Could you check a few things on this drawing? It's one solid part, dimensions in mm from its lowest x, y, z. A direction names the side the tool comes from. Round coordinates to 2 decimals unless told otherwise and drop trailing zeros. Loops run counter-clockwise (first coordinate to the right, second up) from the corner with the lowest first, then second, coordinate; pieces in that order, holes last. Notation, with made-up numbers: (81.5, -11) -> (118.5, -11) arc R31 cw to (118.5, 19) -> close; hole circle Ø7 at (-38.5, 54.25). An arc over 180 degrees is marked (long way). Use CSV: the item, a comma, the result in double quotes. Start each with the question number.
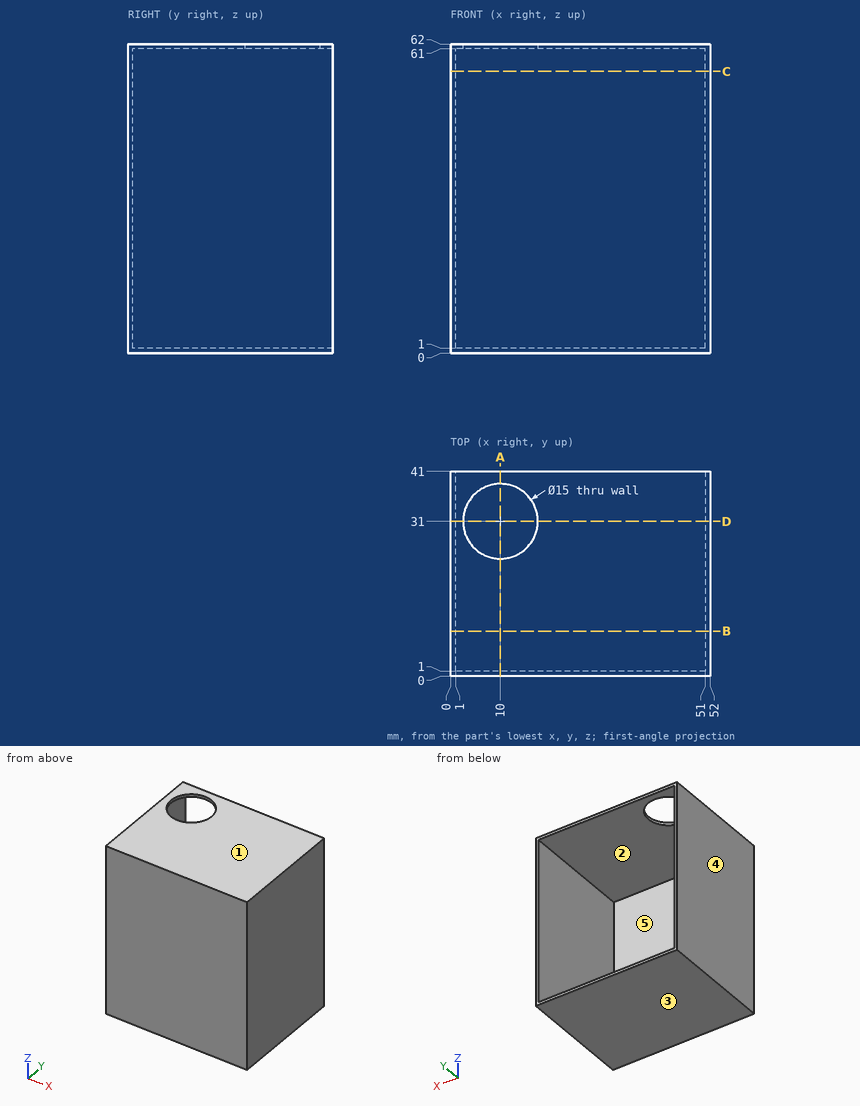
Q1. I want a section at A-A, the plane x = 10. List the corners of the cut face in (y, z) for me.
Q2. For the marked faces 1 and 2, which set-ups out of +Z, -Z, +X, -X, +Y, -Y let a thin tool reach every point of the face, with its end or its side?
Q3. I want a section at C-C, the plane z = 56.5. List the corners of the cut face in (x, y) for me.
Q4. I need wall thicknesses on line 1 along X through (y, z) = (9, 40); line 2 along Z through (x, y) = (50.5, 37.5); line 3 along Y through (x, z) = (10, 61.5). Which ranges of each line are inside material? Lowest first, please.
Q5. If we mould it in two halves opening along X, with no side actions, what happens to the marked faces 3, 4 and 5? For each: pulls with the +X half, pulls with the -X half, needs draft (parallel to the pull), parting line crosses it, or undercut.
Q6. I want a section at D-D, the plane y = 31. List the corners of the cut face in (x, z) for me.
Q7. I want a section at B-B, the plane y = 9. List the corners of the cut face in (x, z) for me.
Q8. Will these pins go through, and if not, where does the flat tip stop? pin 1 Ø4 at (x, z) = (7, 17) entering from -Y; pin 2 Ø10 at (x, z) = (21.5, 51.5) entering from +Y.
Values found:
1,outline,"(0, 0) -> (41, 0) -> (41, 1) -> (1, 1) -> (1, 61) -> (23.5, 61) -> (23.5, 62) -> (0, 62) -> close; (38.5, 61) -> (41, 61) -> (41, 62) -> (38.5, 62) -> close"
2,face 1,"+Z, +X, -X, +Y, -Y"
2,face 2,"+Y"
3,outline,"(0, 0) -> (52, 0) -> (52, 41) -> (51, 41) -> (51, 1) -> (1, 1) -> (1, 41) -> (0, 41) -> close"
4,line 1,"0 to 1, 51 to 52"
4,line 2,"0 to 1, 61 to 62"
4,line 3,"0 to 23.5, 38.5 to 41"
5,face 3,"needs draft"
5,face 4,"pulls with the -X half"
5,face 5,"undercut"
6,outline,"(0, 0) -> (52, 0) -> (52, 62) -> (17.5, 62) -> (17.5, 61) -> (51, 61) -> (51, 1) -> (1, 1) -> (1, 61) -> (2.5, 61) -> (2.5, 62) -> (0, 62) -> close"
7,outline,"(0, 0) -> (52, 0) -> (52, 62) -> (0, 62) -> close; hole (1, 1) -> (51, 1) -> (51, 61) -> (1, 61) -> close"
8,pin 1,"y = 0"
8,pin 2,"y = 1"
